Build history of the part. All positions in model axes, mm. Give positions to 0.01 mm unless a question says otherwise; leave off trailing zeros. Order: outer loops, then holes, each group sorted by start corner. A loop starts at its lowest first (then second) coordinate and runs counter-clockwise, first axis right, second up. Notation, with made-up numbers: (-28, 21.25) -> (-23, 21.25) arc R25 ccw to (-23, 45.25) -> close; hole circle Ø1 at (50, 87). An arc over 180 degrees is marked (long way). One line per question, with ' | ' between items. Start each with the question number.
(1) Pin check, flat tips, straight feed: pin 1 Ø5 at (y, z) = (-641, -15.5) entering from +X; pin 2 Ø6 at (x, z) = (541, -15.5) entering from -Y; pin 3 Ø2 at (y, z) = (-333, -8) entering from +X. Stop position of each tip, or through.
(2) Drill centre lines: L1, parallel to Y at x = 500, z = -9.25; L2, parallel to Y at x = 312, z = -14.5; L3, parallel to X at y = -530, z = -2.25. Where is each one in solid material? Low to high. Write a range as from..to.
(3) Cut at C-C (y = -368.5). Give the cut face in (x, z), then the cut area to 3 significant figures.
(4) Cut at B-B (x = 426.5). Give the cut face in (y, z), then the cut area to 3 significant figures.
(5) Cut at A-A (z = -21.25). Give the cut face in (x, y) (1 decimal).
Autodesk Inventor part; units mm, degrees
ref_plane "YZ Plane" through (0, 0, 0) normal (1, 0, 0) x (0, 1, 0)
ref_plane "XZ Plane" through (0, 0, 0) normal (0, 1, 0) x (-1, 0, 0)
ref_plane "XY Plane" through (0, 0, 0) normal (0, 0, 1) x (1, 0, 0)
sketch "Sketch1" plane through (0, 0, 0) normal (0, 0, 1) x (1, 0, 0)
  line L0 (-18.0719, 15.5659) -> (782.0281, 15.5659) construction
  line L1 (782.0281, 15.5659) -> (782.0281, -1051.2341) construction
  line L2 (782.0281, -1051.2341) -> (-18.0719, -1051.2341) construction
  line L3 (-18.0719, -1051.2341) -> (-18.0719, 15.5659) construction
  line L4 (450.0641, -291.2392) -> (533.9512, -409.0865)
  line L5 (533.9512, -409.0865) -> (533.9512, -496.2541)
  line L6 (533.9512, -496.2541) -> (556.2067, -578.785)
  line L7 (556.2067, -578.785) -> (576.8305, -655.2648)
  line L8 (576.8305, -655.2648) -> (554.4974, -746.6723)
  line L9 (554.4974, -746.6723) -> (443.3726, -760.9041)
  line L10 (443.3726, -760.9041) -> (297.7206, -756.0491)
  line L11 (297.7206, -756.0491) -> (235.4159, -678.9444)
  line L12 (235.4159, -678.9444) -> (255.9915, -400.8879)
  line L13 (255.9915, -400.8879) -> (284.4547, -276.0204)
  line L14 (284.4547, -276.0204) -> (450.0641, -291.2392)
  line L15 (576.8305, -760.9041) -> (235.4159, -760.9041)
  line L16 (235.4159, -760.9041) -> (235.4159, -276.0204)
  line L17 (235.4159, -276.0204) -> (576.8305, -276.0204)
  line L18 (576.8305, -276.0204) -> (576.8305, -760.9041)
  point P0 (0, 0)
  dimension "d7" = 341.4146
  dimension "d10" = 484.8837
extrude "Extrusion1" add sketch "Sketch1" against normal blind 25.4 contours L4 L5 L6 L7 L8 L9 L10 L11 L12 L13 L14
properties part number "bingo"
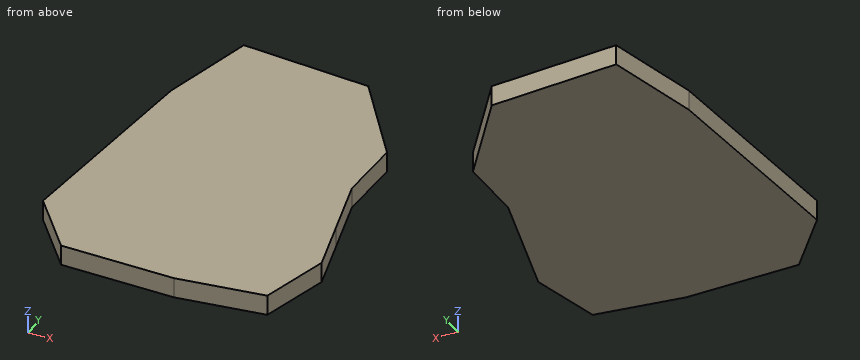
Result set:
1) pin 1: stops at x = 573.66 | pin 2: stops at y = -748.79 | pin 3: stops at x = 480.5
2) L1: y = -753.65..-361.39 | L2: y = -756.53..-278.55 | L3: x = 246.44..543.05
3) outline: (263.37, -25.4) -> (505.06, -25.4) -> (505.06, 0) -> (263.37, 0) -> close | area: 6,140 mm2
4) outline: (-760.34, -25.4) -> (-289.07, -25.4) -> (-289.07, 0) -> (-760.34, 0) -> close | area: 12,000 mm2
5) outline: (235.4, -678.9) -> (297.7, -756) -> (443.4, -760.9) -> (554.5, -746.7) -> (576.8, -655.3) -> (556.2, -578.8) -> (534, -496.3) -> (534, -409.1) -> (450.1, -291.2) -> (284.5, -276) -> (256, -400.9) -> close
